Verification items for the finished model (mm, model axes). Face numbers are marked on the shaded views. A direction names the side the tool comes from. Round coordinates to 2 decimals unless told otherwise and drop trailing zeros. Write each loop counter-clockwise with the first axis right and the second up, starting at its lowest first coordinate (ties: lowest second). Pieces come first, ordered by that corner, then holes. Notation, with made-up numbers: M 16.25,14 L 42.25,14 A27 cw 42.25,43 Z; hole C 11.5,50.5 d4. An arc over 180 degrees is marked long. Write each question's results on one line, items separated by ' | '.
from build123d import *

# Parameters (mm, degrees)
BOSS_EXTRUDE1_DEPTH = 250


with BuildPart() as part:
    # Sketch1 → Boss-Extrude1 (new body, symmetric)
    with BuildSketch(Plane(origin=(0, 0, 0), x_dir=(0, 0, -1), z_dir=(1, 0, 0))):
        Polygon((-33.959336145, 53.010184438), (16.040663855, 53.010184438), (16.040663855, -16.989815562), (-33.959336145, -16.989815562), (-33.959336145, -11.989815562), (11.040663855, -11.989815562), (11.040663855, 48.010184438), (-33.959336145, 48.010184438), align=None)
    extrude(amount=BOSS_EXTRUDE1_DEPTH, both=True)


solid = part.part
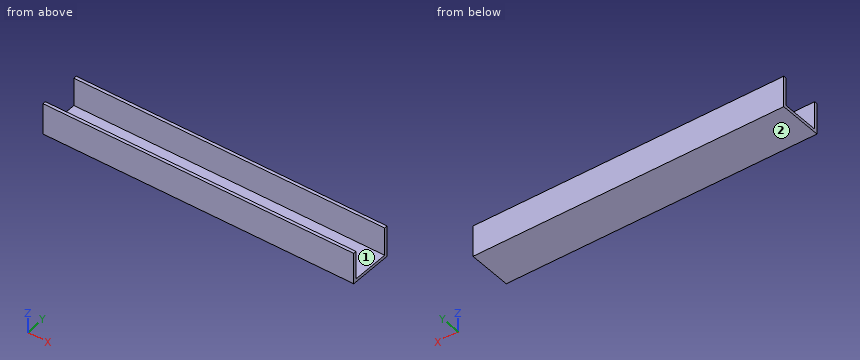
1) Access from +Z, -Z, +X, -X, +Y, -Y to the whole of each face (thin tool, end or side, straight path). Record for the marked faces 1 and 2.
Calculated:
face 1: +Z, +X, -X | face 2: -Z, +X, -X, +Y, -Y
2) Material ranges on line 1 (Y direction, x = -149, z = 1.5); line 2 (Z direction, x = -72, y = 32.5), recorded low to high. Write a range as [from, to].
Calculated:
line 1: y = [-16.99, -11.99], [48.01, 53.01] | line 2: z = [-16.04, -11.04]
3) Depth check by flat-ended pin: P1, Ø1, axis at x = 111, y = -2, coming from the +Z side. Enter the tip coordinate at first touch or a pass-through.
Calculated:
P1: stops at z = -11.04
4) Sectioned sample at A-A, the plane z = 4.5. Record the cut outline in (x, y).
Calculated:
outline: M -250,-16.99 L 250,-16.99 L 250,-11.99 L -250,-11.99 Z; M -250,48.01 L 250,48.01 L 250,53.01 L -250,53.01 Z
5) Sectioned sample at C-C, the plane y = 34.5. Record the cut outline in (x, z).
Calculated:
outline: M -250,-16.04 L 250,-16.04 L 250,-11.04 L -250,-11.04 Z
6) Sectioned sample at B-B, the plane x = -201.5. Record the cut outline in (y, z).
Calculated:
outline: M -16.99,-16.04 L 53.01,-16.04 L 53.01,33.96 L 48.01,33.96 L 48.01,-11.04 L -11.99,-11.04 L -11.99,33.96 L -16.99,33.96 Z
